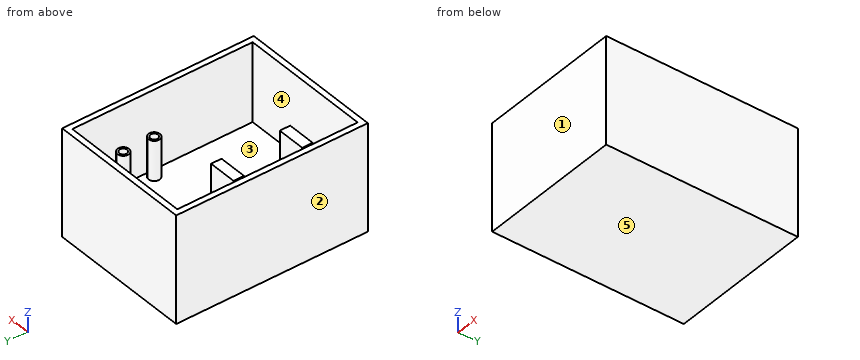
```python
from build123d import *

# Parameters (mm, degrees)
SKETCH1_W                 = 64.4906
SKETCH1_H                 = 86.0806
SKETCH1_W_2               = 59.4106
SKETCH1_H_2               = 81.0006
EXTRUDE_THIN1_DEPTH       = 35.3568
SKETCH2_W                 = 64.4906
SKETCH2_H                 = 86.0806
BOSS_EXTRUDE1_DEPTH       = 12.7
SKETCH3_W                 = 12.7
SKETCH3_H                 = 4.692408937
BOSS_EXTRUDE3_DEPTH       = 12.7
BOSS_EXTRUDE4_DEPTH       = 17.78
F_8_32_TAPPED_HOLE1_D     = 3.4544
F_8_32_TAPPED_HOLE1_DEPTH = 18.796
F_8_32_TAPPED_HOLE1_TIP   = 1.037806461


with BuildPart() as part:
    # Sketch1 → Extrude-Thin1 (new body)
    with BuildSketch(Plane.XY):
        Rectangle(SKETCH1_W, SKETCH1_H)
        Rectangle(SKETCH1_W_2, SKETCH1_H_2, mode=Mode.SUBTRACT)
    extrude(amount=EXTRUDE_THIN1_DEPTH)

    # Sketch2 → Boss-Extrude1 (add)
    with BuildSketch(Plane(origin=(0, 0, 0), x_dir=(-1, 0, 0), z_dir=(0, 0, -1))):
        Rectangle(SKETCH2_W, SKETCH2_H)
    extrude(amount=BOSS_EXTRUDE1_DEPTH)

    # Sketch3 → Boss-Extrude3 (add)
    with BuildSketch(Plane.XY):
        with Locations((0.486291995, -6.023095532)):
            Rectangle(SKETCH3_W, SKETCH3_H)
        with Locations((0.486291995, -36.877504469)):
            Rectangle(SKETCH3_W, SKETCH3_H)
    extrude(amount=BOSS_EXTRUDE3_DEPTH)

    # Sketch5 → Boss-Extrude4 (add)
    with BuildSketch(Plane.XY):
        with BuildLine():
            Line((-26.393952246, 7.409416617), (-26.393952246, 4.869416617))
            Line((-26.393952246, 4.869416617), (-23.853952246, 4.869416617))
            ThreePointArc((-23.853952246, 4.869416617), (-24.597901022, 6.665467841), (-26.393952246, 7.409416617))
        make_face()
        with BuildLine():
            Line((-23.853952246, 4.869416617), (-26.393952246, 4.869416617))
            Line((-26.393952246, 4.869416617), (-26.393952246, 7.409416617))
            ThreePointArc((-26.393952246, 7.409416617), (-28.19000347, 3.073365392), (-23.853952246, 4.869416617))
        make_face()
        with BuildLine():
            ThreePointArc((-23.853952246, 35.630883383), (-28.19000347, 37.426934608), (-26.393952246, 33.090883383))
            Line((-26.393952246, 33.090883383), (-26.393952246, 35.630883383))
            Line((-26.393952246, 35.630883383), (-23.853952246, 35.630883383))
        make_face()
        with BuildLine():
            Line((-26.393952246, 35.630883383), (-26.393952246, 33.090883383))
            ThreePointArc((-26.393952246, 33.090883383), (-24.597901022, 33.834832159), (-23.853952246, 35.630883383))
            Line((-23.853952246, 35.630883383), (-26.393952246, 35.630883383))
        make_face()
        with BuildLine():
            ThreePointArc((26.393952246, 22.79015), (23.853952246, 20.25015), (26.393952246, 17.71015))
            Line((26.393952246, 17.71015), (26.393952246, 22.79015))
        make_face()
        with BuildLine():
            Line((26.393952246, 22.79015), (26.393952246, 17.71015))
            ThreePointArc((26.393952246, 17.71015), (28.19000347, 18.454098776), (28.933952246, 20.25015))
            ThreePointArc((28.933952246, 20.25015), (28.19000347, 22.046201224), (26.393952246, 22.79015))
        make_face()
        with BuildLine():
            ThreePointArc((26.393952246, 8.878390919), (24.137539747, 7.504668174), (24.321824233, 4.869416617))
            Line((24.321824233, 4.869416617), (26.393952246, 4.869416617))
            Line((26.393952246, 4.869416617), (26.393952246, 8.878390919))
        make_face()
        with BuildLine():
            Line((26.393952246, 4.869416617), (24.321824233, 4.869416617))
            ThreePointArc((24.321824233, 4.869416617), (27.164794269, 3.918183784), (28.933952246, 6.338390919))
            ThreePointArc((28.933952246, 6.338390919), (28.19000347, 8.134442143), (26.393952246, 8.878390919))
            Line((26.393952246, 8.878390919), (26.393952246, 4.869416617))
        make_face()
    extrude(amount=BOSS_EXTRUDE4_DEPTH)

    # #8-32 Tapped Hole1
    with Locations(Plane(origin=(-26.393952246, 4.869416617, 17.78), x_dir=(1, 0, 0), z_dir=(0, 0, 1))):
        with Locations((0, 0), (0, 30.761466766), (52.787904492, 15.380733383), (52.787904492, 1.468974302)):
            Hole(F_8_32_TAPPED_HOLE1_D / 2, depth=F_8_32_TAPPED_HOLE1_DEPTH)
            with Locations((0, 0, -(F_8_32_TAPPED_HOLE1_DEPTH + F_8_32_TAPPED_HOLE1_TIP / 2))):  # 118° drill point
                Cone(0, F_8_32_TAPPED_HOLE1_D / 2, F_8_32_TAPPED_HOLE1_TIP, mode=Mode.SUBTRACT)


solid = part.part
```
Geometry check sheet. Reference: the model listing, model coordinates, mm. Face numbers are marked on the shaded views. A direction names the side the tool comes from. Give positions to 0.01 mm unless a question says otherwise; leave off trailing zeros. Write each loop counter-clockwise with the first axis right and the second up, starting at its lowest first coordinate (ties: lowest second). Pieces come first, ordered by that corner, then holes.
1) Section check C-C, the plane x = -2.5. Record the boundary of the cut face in (y, z).
2) Material ranges on L1, parallel to X at y = 35.5, z = 5; L2, parallel to X at y = 20, z = 10.5; L3, parallel to X at y = -21, z = 6.5, recorded low to high.
3) Gauge pin test, flat ends, axial feed: pin 1 (5 mm diameter, centred on x = 1.5, y = -36, fed in from +Z); pin 2 (4 mm diameter, centred on x = 26.39, y = 6.34, fed in from +Z); pin 3 (1 mm diameter, centred on x = -18, y = -32.5, fed in from +Z). Record the tip position at first contact, or that the pin passes through.
4) Section check D-D, the plane y = 10.5. Record the boundary of the cut face in (x, z), and give its area (3 significant figures).
5) Section check A-A, the plane z = 2. State how many separate pieces and enclosed holes the cut face has, and give its area (3 significant figures).
6) Access from +Z, -Z, +X, -X, +Y, -Y to the whole of each face (thin tool, end or side, straight path). Record for the marked faces 4 and 5.
7) Release check for a two-part mould opening along Y. For the marked faces 1, 2 and 3 record: pulls with the +Y half, pulls with the -Y half, needs draft (parallel to the pull), parting line crosses it, or undercut.
Computed:
1. outline: (-43.04, -12.7) - (43.04, -12.7) - (43.04, 35.36) - (40.5, 35.36) - (40.5, 0) - (-3.68, 0) - (-3.68, 12.7) - (-8.37, 12.7) - (-8.37, 0) - (-34.53, 0) - (-34.53, 12.7) - (-39.22, 12.7) - (-39.22, 0) - (-40.5, 0) - (-40.5, 35.36) - (-43.04, 35.36) - close
2. L1: x = -32.25 to -29.71, -28.93 to -28.12, -24.67 to -23.86, 29.71 to 32.25
2. L2: x = -32.25 to -29.71, 23.87 to 24.68, 28.1 to 28.92, 29.71 to 32.25
2. L3: x = -32.25 to -29.71, 29.71 to 32.25
3. pin 1: stops at z = 12.7
3. pin 2: stops at z = 17.78
3. pin 3: stops at z = 0
4. outline: (-32.25, -12.7) - (32.25, -12.7) - (32.25, 35.36) - (29.71, 35.36) - (29.71, 0) - (-29.71, 0) - (-29.71, 35.36) - (-32.25, 35.36) - close
4. area: 999 mm2
5. separate pieces: 7
5. enclosed holes: 5
5. area: 902 mm2
6. face 4: +Z
6. face 5: -Z, +X, -X, +Y, -Y
7. face 1: pulls with the -Y half
7. face 2: needs draft
7. face 3: undercut
